from build123d import *

# Parameters (mm, degrees)
SKETCH_1_R          = 1.45
EXTRUDE_1_DEPTH     = 3
EXTRUDE_2_DEPTH     = 3
SKETCH_4_W          = 40
SKETCH_4_H          = 55
CUT_EXTRUDE_2_DEPTH = 73.734104793
SKETCH_5_W          = 15
SKETCH_5_H          = 22
EXTRUDE_3_DEPTH     = 3
SKETCH_6_W          = 10
SKETCH_6_H          = 7.1
CUT_EXTRUDE_3_DEPTH = 73.734104793
FILLET_1_R          = 2
FILLET_2_R          = 1.5


with BuildPart() as part:
    # 草图1 → 凸台-拉伸1 (new body)
    with BuildSketch(Plane(origin=(0, 0, 0), x_dir=(1, 0, 0), z_dir=(0, 1, 0))):
        Polygon((-47.5, 0), (0, 0), (47.5, 0), (47.5, -15), (7.5, -15), (7.5, -55), (-7.5, -55), (-7.5, -15), (-47.5, -15), align=None)
        with Locations(Location((0, -7.5, 0), (0, 0, 270))):
            Circle(SKETCH_1_R, mode=Mode.SUBTRACT)
        with Locations(Location((0, -30, 0), (0, 0, 270))):
            Circle(SKETCH_1_R, mode=Mode.SUBTRACT)
        with Locations(Location((0, -50, 0), (0, 0, 270))):
            Circle(SKETCH_1_R, mode=Mode.SUBTRACT)
        with Locations(Location((-22.5, -7.5, 0), (0, 0, 270))):
            Circle(SKETCH_1_R, mode=Mode.SUBTRACT)
        with Locations(Location((-42.5, -7.5, 0), (0, 0, 270))):
            Circle(SKETCH_1_R, mode=Mode.SUBTRACT)
        with Locations(Location((42.5, -7.5, 0), (0, 0, 90))):
            Circle(SKETCH_1_R, mode=Mode.SUBTRACT)
        with Locations(Location((22.5, -7.5, 0), (0, 0, 90))):
            Circle(SKETCH_1_R, mode=Mode.SUBTRACT)
    extrude(amount=EXTRUDE_1_DEPTH)

    # 草图2 → 凸台-拉伸2 (add)
    with BuildSketch(Plane(origin=(0, 3, 0), x_dir=(1, 0, 0), z_dir=(0, 1, 0))):
        Polygon((-47.5, -15), (-7.5, -55), (-7.5, -45.100505063), (-37.600505063, -15), align=None)
        Polygon((37.600505063, -15), (47.5, -15), (7.5, -55), (7.5, -45.100505063), align=None)
    extrude(amount=-EXTRUDE_2_DEPTH)

    # 草图4 → 切除-拉伸2 (cut, through all)
    with BuildSketch(Plane(origin=(0, 3, 0), x_dir=(1, 0, 0), z_dir=(0, 1, 0))):
        with Locations((27.5, -27.5)):
            Rectangle(SKETCH_4_W, SKETCH_4_H)
    extrude(amount=-CUT_EXTRUDE_2_DEPTH, mode=Mode.SUBTRACT)

    # 草图5 → 凸台-拉伸3 (add)
    with BuildSketch(Plane(origin=(0, 3, 0), x_dir=(1, 0, 0), z_dir=(0, 1, 0))):
        with Locations((0, 11)):
            Rectangle(SKETCH_5_W, SKETCH_5_H)
    extrude(amount=-EXTRUDE_3_DEPTH)

    # 草图6 → 切除-拉伸3 (cut, through all)
    with BuildSketch(Plane(origin=(0, 3, 0), x_dir=(1, 0, 0), z_dir=(0, 1, 0))):
        with Locations((0, 18.45)):
            Rectangle(SKETCH_6_W, SKETCH_6_H)
    extrude(amount=-CUT_EXTRUDE_3_DEPTH, mode=Mode.SUBTRACT)

    # 圆角1
    fillet_1_edges = [part.edges().sort_by_distance(p)[0] for p in [
        (-7.5, 1.5, 0),
        (-5, 1.5, -14.9),
        (5, 1.5, -14.9),
        (-47.5, 1.5, 0),
        (7.5, 1.5, 55),
        (-7.5, 1.5, 55),
        (-7.5, 1.5, 15),
        (-47.5, 1.5, 15),
        (-7.5, 1.5, 45.100505063),
        (-37.600505063, 1.5, 15),
    ]]
    fillet(fillet_1_edges, radius=FILLET_1_R)

    # 圆角2
    fillet_2_edges = [part.edges().sort_by_distance(p)[0] for p in [
        (-5, 1.5, -22),
        (5, 1.5, -22),
    ]]
    fillet(fillet_2_edges, radius=FILLET_2_R)


solid = part.part
Can you work these out from the model? Positions are in its coordinate system, mm. A direction names the side the tool comes from. Give positions to 0.01 mm unless a question says otherwise; leave off trailing zeros. Write each loop counter-clockwise with the first axis right and the second up, starting at its lowest first coordinate (ties: lowest second). Pieces come first, ordered by that corner, then holes. Notation, with made-up numbers: M 58.25,74 L 75.25,74 A14 cw 75.25,101 Z; hole C 28,9.25 d10. An arc over 180 degrees is marked long. Answer in a Markdown table with one row per item. Add a question column.
Item 1: Imagine slicing it at A-A, the plane x = 0. Write out the boundary of the cut face in (y, z), plus the area to 3 significant figures.
Item 2: Please list where these lines run through material, in increasing order: L1, parallel to X at y = 0.9, z = 7.5; L2, parallel to X at y = 2.75, z = -17; L3, parallel to Z at x = -29.5, y = 2.25.
Item 3: Imagine slicing it at C-C, the plane z = 7.5. Write out the boundary of the cut face in (x, y), plus the area to 3 significant figures.
Item 4: On a 3-axis mill with a long thin cutter (end or side, diameter ignored), from which of +Z, -Z, +X, -X, +Y, -Y can I reach the whole of each face in a straight line? I mean faces 5 (the flat face through (-2, 0, 25)), 6 (the flat face through (-2, 3, 25)), 7 (the cylindrical face through (-34.632, 1.479, 16.265)), 8 (the flat face through (0, 2, -14.9)), 9 (the flat face through (-7.5, 2, -12)). Say none if no direction works.
Item 5: We'd pull the mould along X, two halves only. Please class faces 1 (the flat face through (-47.5, 1, 8)), 2 (the cylindrical face through (6.93, 1.52, 54.4)), 3 (the cylindrical face through (-8.07, 1.52, 15.6)), 4 (the flat face through (-5, 2, -19)): released by +X, released by -X, zero draft, split by the parting line, or undercut.
Item 6: Imagine slicing it at B-B, the plane x = -42.5. Write out the boundary of the cut face in (y, z).
Item 7: Imagine slicing it at D-D, the plane y = 0.6. State how many separate pieces and enclosed holes the cut face has, plus the area to 3 significant figures.
Item 8: For pin 1 Ø0.9 at (y, z) = (1, -18) entering from -X; pin 2 Ø1.5 at (x, y) = (-25, 1.5) entering from +Z; pin 3 Ø4 at (x, z) = (0, 30) entering from +Y; pin 4 Ø1.5 at (x, y) = (-31.5, 2) entering from -Z, each with a flat end and sliding along its axis, tell me the tip position at first contact or that it passes through.
Evaluation:
| question | item | result |
|---|---|---|
| 1 | outline | M 0,-14.9 L 3,-14.9 L 3,6.05 L 0,6.05 Z; M 0,8.95 L 3,8.95 L 3,28.55 L 0,28.55 Z; M 0,31.45 L 3,31.45 L 3,48.55 L 0,48.55 Z; M 0,51.45 L 3,51.45 L 3,55 L 0,55 Z |
| 1 | area | 184 mm² |
| 2 | L1 | x = -47.5 to -43.95, -41.05 to -23.95, -21.05 to -1.45, 1.45 to 7.5 |
| 2 | L2 | x = -7.5 to -5, 5 to 7.5 |
| 2 | L3 | z = 0 to 15, 23.1 to 33 |
| 3 | outline | M -47.5,0 L -43.95,0 L -43.95,3 L -47.5,3 Z; M -41.05,0 L -23.95,0 L -23.95,3 L -41.05,3 Z; M -21.05,0 L -1.45,0 L -1.45,3 L -21.05,3 Z; M 1.45,0 L 7.5,0 L 7.5,3 L 1.45,3 Z |
| 3 | area | 139 mm² |
| 4 | face 5 | +Z, -Z, +X, -X, -Y |
| 4 | face 6 | +Z, -Z, +X, -X, +Y |
| 4 | face 7 | +Y, -Y |
| 4 | face 8 | -Z, +Y, -Y |
| 4 | face 9 | -Z, -X, +Y, -Y |
| 5 | face 1 | released by -X |
| 5 | face 2 | released by +X |
| 5 | face 3 | undercut |
| 5 | face 4 | undercut |
| 6 | outline | M 0,0 L 3,0 L 3,6.05 L 0,6.05 Z; M 0,8.95 L 3,8.95 L 3,20 L 0,20 Z |
| 7 | separate pieces | 1 |
| 7 | enclosed holes | 6 |
| 7 | area | 2,010 mm² |
| 8 | pin 1 | stops at x = -7.5 |
| 8 | pin 2 | stops at z = 38.25 |
| 8 | pin 3 | stops at y = 3 |
| 8 | pin 4 | stops at z = 0 |
